from build123d import *

# Parameters (mm, degrees)
F0_W     = 79
F0_H     = 24.5
F1_DEPTH = 3.2
F2_W     = 99.5
F2_H     = 44.5
F3_DEPTH = 2
F4_R     = 12
F4_R_2   = 1.5
F5_DEPTH = 5.2


with BuildPart() as f1:
    # F0 (on Top) → F1 (new body)
    with BuildSketch(Plane.XY):
        Rectangle(F0_W, F0_H)
    extrude(amount=F1_DEPTH)

    # F2 (on face) → F3 (join)
    with BuildSketch(Plane.XY.offset(3.2)):
        Rectangle(F2_W, F2_H)
    extrude(amount=F3_DEPTH)

    # F4 (on face) → F5 (cut, through all)
    with BuildSketch(Plane.XY.offset(5.2)):
        Circle(F4_R)
        with Locations((-15.25, 0)):
            Circle(F4_R_2)
        with Locations((15.25, 0)):
            Circle(F4_R_2)
    extrude(amount=-F5_DEPTH, mode=Mode.SUBTRACT)


solid = f1.part
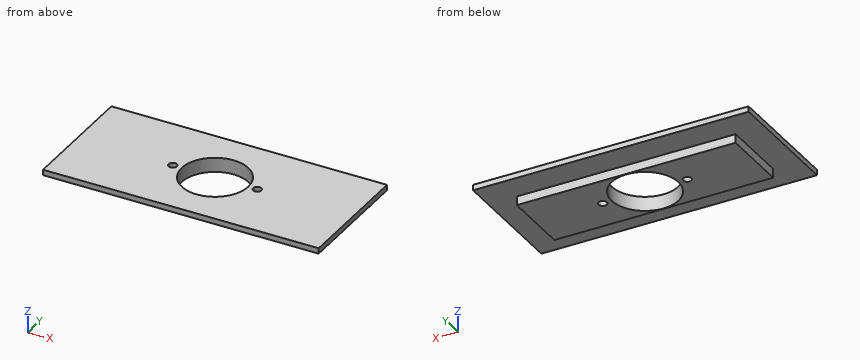
Geometry check sheet. Reference: the model listing, model coordinates, mm. Give positions to 0.01 mm unless a question says otherwise; leave off trailing zeros. Write each loop counter-clockwise with the first axis right and the second up, starting at its lowest first coordinate (ties: lowest second). Pieces come first, ordered by that corner, then holes. Notation, with made-up numbers: M 56.5,22.25 L 93.5,22.25 A28 cw 93.5,47.25 Z; hole C 85.5,80 d6. An arc over 180 degrees is marked long. Answer as CSV lines item,"result". Start each with the question number.
Q1. Go/stop test with flat-tipped pins: pin 1 (1.6 mm diameter, centred on x = 8, z = 2, fed in from -Y); pin 2 (1 mm diameter, centred on y = 5, z = 1, fed in from -X); pin 3 (1 mm diameter, centred on y = -3.5, z = 1, fed in from +X); pin 4 (14.5 mm diameter, centred on x = 0, y = 0, fed in from -Z). Record where each tip stops, or that it passes through.
Q2. Section check C-C, the plane y = -6.5. Record the cut outline in (x, z).
Q3. Section check A-A, the plane x = 0. Record the cut outline in (y, z), then the cut area to 3 significant figures.
Q4. Section check B-B, the plane z = 0.9. Record the cut outline in (x, y), then the cut area to 3 significant figures.
Q5. Section check D-D, the plane x = -37.5. Record the cut outline in (y, z).
Q6. Material ranges on L1, parallel to Y at x = -15.25, z = 3.3; L2, parallel to Y at x = -15.25, z = 2.65; L3, parallel to Z at x = -4, y = -14.5, recorded low to high.
Geometry says:
1,pin 1,"y = -12.25"
1,pin 2,"x = -39.5"
1,pin 3,"x = 39.5"
1,pin 4,"through"
2,outline,"M -49.75,3.2 L -39.5,3.2 L -39.5,0 L -10.09,0 L -10.09,5.2 L -49.75,5.2 Z; M 10.09,0 L 39.5,0 L 39.5,3.2 L 49.75,3.2 L 49.75,5.2 L 10.09,5.2 Z"
3,outline,"M -22.25,3.2 L -12.25,3.2 L -12.25,0 L -12,0 L -12,5.2 L -22.25,5.2 Z; M 12,0 L 12.25,0 L 12.25,3.2 L 22.25,3.2 L 22.25,5.2 L 12,5.2 Z"
3,area,"42.6 mm^2"
4,outline,"M -39.5,-12.25 L 39.5,-12.25 L 39.5,12.25 L -39.5,12.25 Z; hole C -15.25,0 d3; hole C 0,0 d24; hole C 15.25,0 d3"
4,area,"1,470 mm^2"
5,outline,"M -22.25,3.2 L -12.25,3.2 L -12.25,0 L 12.25,0 L 12.25,3.2 L 22.25,3.2 L 22.25,5.2 L -22.25,5.2 Z"
6,L1,"-22.25 to -1.5, 1.5 to 22.25"
6,L2,"-12.25 to -1.5, 1.5 to 12.25"
6,L3,"3.2 to 5.2"
